Here's how the part is built. I have some questions about the finished solid (model axes, mm). A direction names the side the tool comes from. Give positions to 0.01 mm unless a question says otherwise; leave off trailing zeros. Loops run counter-clockwise (first coordinate to the right, second up) from the corner with the lowest first, then second, coordinate; pieces in that order, holes last.
Q1. I need wall thicknesses on probe 1 along X at (y, z) = (0, 10.95); probe 2 along Y at (x, z) = (0, 10.65); probe 3 along Z at (x, y) = (-15, -25.5). Which ranges of each line are inside material? Lowest first, please.
Q2. For faces 1 (the face through (-8, 18, 9.5)), 2 (the face through (-18, -28, 0)), 3 (the face through (-23.451, -26.105, -0.182)), which set-ups out of +Z, -Z, +X, -X, +Y, -Y let a thin tool reach every point of the face, with its end or its side?
Q3. Suppose I cut it at A-A (x = 0). List the corners of the cut face in (y, z) for me.
Q4. Suppose I cut it at C-C (z = -6). List the corners of the cut face in (x, y) for me, and give its area (3 significant figures).
Q5. Suppose I cut it at D-D (x = 10.5). List the corners of the cut face in (y, z) for me.
Q6. I'm going to push flat-ended pins straight in: P1, Ø23, axis at x = 0, y = 0, coming from the -Z side; P2, Ø2, axis at x = 22, z = -1, coming from the +Y side; P3, Ø13, axis at y = 0, z = 3, coming from the +X side; P4, Ø5, axis at x = 15, z = 0, coming from the -Y side. Where does each tip first touch, or does it pass through?
Q7. Thinking about a two-plate mould opening in Y: for faces 4 (the face through (15.02, 24.02, -0.18)), 5 (the face through (27, -5, 0)), 6 (the face through (-14.5, -22, 0)), 7 (the face through (-8, 18, -9.5)), which applies, pulls with the +Y half, pulls with the -Y half, needs draft (parallel to the pull), parting line crosses it, or undercut?
Q8. Suppose I cut it at B-B (y = -3). List the corners of the cut face in (x, z) for me, and give its area (3 significant figures).
```python
from build123d import *

# Parameters (mm, degrees)
BOSS_EXTRUDE1_DEPTH          = 13
CUT_EXTRUDE1_DEPTH           = 9.5
CUT_EXTRUDE1_DEPTH_BACK      = 9.5
SKETCH2_R                    = 21.5
CUT_EXTRUDE2_REACH           = 71.399
CUT_EXTRUDE2_END_RADIUS      = 21.5
SKETCH3_R                    = 9
F_6_0_6_DIAMETER_HOLE1_D     = 6
F_6_0_6_DIAMETER_HOLE1_DEPTH = 10
F_6_0_6_DIAMETER_HOLE1_TIP   = 1.802581857


with BuildPart() as part:
    # Sketch1 → Boss-Extrude1 (new, symmetric)
    with BuildSketch(Plane(origin=(0, 0, 0), x_dir=(-1, 0, 0), z_dir=(0, 0, -1))):
        with BuildLine():
            Line((-27, 7.5), (-27, -18.5))
            Line((-27, -18.5), (-20, -33.5))
            Line((-20, -33.5), (20, -33.5))
            Line((20, -33.5), (27, -18.5))
            Line((27, -18.5), (27, -15.5))
            Line((27, -15.5), (27, 2))
            ThreePointArc((27, 2), (20.263455967, 18.263455967), (4, 25))
            Line((4, 25), (-8.37877555, 25))
            ThreePointArc((-8.37877555, 25), (-15.10867012, 23.993374436), (-21.249479132, 21.061610355))
            ThreePointArc((-21.249479132, 21.061610355), (-34.365218355, 18.623068776), (-27, 7.5))
        make_face()
        with BuildLine():
            ThreePointArc((-16.651259459, 9.559056356), (-9.559056356, -16.651259459), (16.651259459, -9.559056356))
            ThreePointArc((16.651259459, -9.559056356), (9.559056356, 16.651259459), (-16.651259459, 9.559056356))
        make_face(mode=Mode.SUBTRACT)
    extrude(amount=BOSS_EXTRUDE1_DEPTH, both=True)

    # Sketch2 → Cut-Extrude1 (cut, two sides: drawn at the far end of the back side and taken through both)
    with BuildSketch(Plane.XY.offset(-CUT_EXTRUDE1_DEPTH_BACK)):
        Circle(SKETCH2_R)
    extrude(amount=CUT_EXTRUDE1_DEPTH + CUT_EXTRUDE1_DEPTH_BACK, mode=Mode.SUBTRACT)

    # Cut-Extrude2: up to this cylinder (the profile starts outside it)
    cut_extrude2_end = Plane(origin=(0, 0, 0), z_dir=(0, 0, -1)) * Cylinder(CUT_EXTRUDE2_END_RADIUS, 186.798, mode=Mode.PRIVATE)
    # Sketch3 → Cut-Extrude2 (cut, up to the surface)
    with BuildSketch(Plane.XZ.offset(33.5), mode=Mode.PRIVATE) as cut_extrude2_sk1:
        with Locations(Location((0, 0, 0), (0, 0, 270))):
            Circle(SKETCH3_R)
    cut_extrude2_tool1 = extrude(cut_extrude2_sk1.sketch, amount=-CUT_EXTRUDE2_REACH, mode=Mode.PRIVATE) - cut_extrude2_end
    add(cut_extrude2_tool1.solids().sort_by_distance((0, -33.5, 0))[0], mode=Mode.SUBTRACT)

    # Ø6.0 (6) Diameter Hole1
    with Locations(Plane(origin=(0, -33.5, 0), x_dir=(-1, 0, 0), z_dir=(0, -1, 0))):
        with Locations((-15, 0), (15, 0)):
            Hole(F_6_0_6_DIAMETER_HOLE1_D / 2, depth=F_6_0_6_DIAMETER_HOLE1_DEPTH)
            with Locations((0, 0, -(F_6_0_6_DIAMETER_HOLE1_DEPTH + F_6_0_6_DIAMETER_HOLE1_TIP / 2))):  # 118° drill point
                Cone(0, F_6_0_6_DIAMETER_HOLE1_D / 2, F_6_0_6_DIAMETER_HOLE1_TIP, mode=Mode.SUBTRACT)


solid = part.part
```
Solutions:
1. probe 1: x = -27 to -19.2, 19.2 to 27
1. probe 2: y = -33.5 to -19.2, 19.2 to 25
1. probe 3: z = -13 to -3, 3 to 13
2. face 1: none
2. face 2: -Y
2. face 3: +Z, -Z, -X, -Y
3. outline: (-33.5, -13) - (-19.2, -13) - (-19.2, -9.5) - (-21.5, -9.5) - (-21.5, -9) - (-33.5, -9) - close; (-33.5, 9) - (-21.5, 9) - (-21.5, 9.5) - (-19.2, 9.5) - (-19.2, 13) - (-33.5, 13) - close; (19.2, -13) - (25, -13) - (25, 13) - (19.2, 13) - (19.2, 9.5) - (21.5, 9.5) - (21.5, -9.5) - (19.2, -9.5) - close
4. outline: (-27, -18.5) - (-20, -33.5) - (-6.71, -33.5) - (-6.71, -20.43) arc R21.5 cw (long way) to (6.71, -20.43) - (6.71, -33.5) - (20, -33.5) - (27, -18.5) - (27, 7.5) arc R8 ccw (long way) to (21.25, 21.06) arc R23 ccw to (8.38, 25) - (-4, 25) arc R23 ccw to (-27, 2) - close
4. area: 1,390 mm2
5. outline: (-33.5, -13) - (-16.07, -13) - (-16.07, -9.5) - (-18.76, -9.5) - (-18.76, 9.5) - (-16.07, 9.5) - (-16.07, 13) - (-33.5, 13) - close; (16.07, -13) - (24.9, -13) - (24.9, 13) - (16.07, 13) - (16.07, 9.5) - (18.76, 9.5) - (18.76, -9.5) - (16.07, -9.5) - close
6. P1: passes through
6. P2: stops at y = 22.43
6. P3: stops at x = 27
6. P4: stops at y = -23.2
7. face 4: pulls with the +Y half
7. face 5: needs draft
7. face 6: pulls with the -Y half
7. face 7: undercut
8. outline: (-27, -13) - (-18.96, -13) - (-18.96, -9.5) - (-21.29, -9.5) - (-21.29, 9.5) - (-18.96, 9.5) - (-18.96, 13) - (-27, 13) - close; (18.96, -13) - (27, -13) - (27, 13) - (18.96, 13) - (18.96, 9.5) - (21.29, 9.5) - (21.29, -9.5) - (18.96, -9.5) - close
8. area: 329 mm2
